```python
from build123d import *

# Parameters (mm, degrees)
BOSS_EXTRUDE1_DEPTH = 9.525
SKETCH2_R           = 10
BOSS_EXTRUDE2_DEPTH = 6.35
CUT_EXTRUDE1_REACH  = 36.757
SKETCH3_R           = 3.175
SKETCH4_R           = 3.175
CUT_EXTRUDE2_DEPTH  = 30.053883131


with BuildPart() as part:
    # Sketch1 → Boss-Extrude1 (new, symmetric)
    with BuildSketch(Plane.XY):
        Polygon((-9.525, 12.7), (-9.525, -12.7), (9.525, -12.7), (9.525, 12.7), (4.445, 12.7), (4.445, -7.62), (-4.445, -7.62), (-4.445, 12.7), align=None)
    extrude(amount=BOSS_EXTRUDE1_DEPTH, both=True)

    # Sketch2 → Boss-Extrude2 (add)
    with BuildSketch(Plane.XZ.offset(12.7)):
        with Locations(Location((0, 0, 0), (0, 0, 162.269593739))):
            Circle(SKETCH2_R)
    extrude(amount=BOSS_EXTRUDE2_DEPTH)

    # Sketch3 → Cut-Extrude1 (cut, up to next)
    with BuildSketch(Plane.XZ.offset(19.05), mode=Mode.PRIVATE) as cut_extrude1_sk1:
        Circle(SKETCH3_R)
    cut_extrude1_tool1 = extrude(cut_extrude1_sk1.sketch, amount=-CUT_EXTRUDE1_REACH, mode=Mode.PRIVATE) & part.part
    add(cut_extrude1_tool1.solids().sort_by_distance((0, -19.05, 0))[0], mode=Mode.SUBTRACT)

    # Sketch4 → Cut-Extrude2 (cut, through all)
    with BuildSketch(Plane(origin=(9.525, 0, 0), x_dir=(0, 0, -1), z_dir=(1, 0, 0))):
        with Locations((0, 3.175)):
            Circle(SKETCH4_R)
    extrude(amount=-CUT_EXTRUDE2_DEPTH, mode=Mode.SUBTRACT)


solid = part.part
```
The listing builds one solid part. Answer for the finished solid, in the listing's coordinates (mm). A direction names the side the tool comes from. Round coordinates to 2 decimals unless told otherwise and drop trailing zeros. Order: outer loops, then holes, each group sorted by start corner. A loop starts at its lowest first (then second) coordinate and runs counter-clockwise, first axis right, second up. Notation, with made-up numbers: (67, 76) - (86, 76) arc R33 ccw to (86, 110) - close; hole circle Ø2 at (5.5, 21). An arc over 180 degrees is marked (long way). Put each result on its own line as item: value. Start each with the question number.
(1) Given P1, Ø1.5, axis at y = -10, z = 1.5, coming from the -X side (3 decimals); P2, Ø4, axis at x = 1, z = 1, coming from the -Y side; P3, Ø12, axis at x = 0.5, y = -3, coming from the -Z side (3 decimals); P4, Ø10, axis at y = 5, z = 3.5, coming from the +X side (3 decimals), each flat-ended and moving along its own axis, determine where each tip first touches the part or whether it passes through.
(2) Find section C-C (y = -7). Give the vertices of the cut face in (x, z) (3 decimals), plus the area to 3 significant figures.
(3) Determine the mould class of faces 5 (the cylindrical face through (-0.69, -13.42, -3.1)), 6 (the flat face through (-4.445, 0, 2)), 7 (the flat face through (0, -8, -9.525)) for opening direction Z: released by +Z, released by -Z, zero draft, split by the parting line, or undercut.
(4) Find section A-A (x = 0). Give the vertices of the cut face in (y, z) (3 decimals), plus the area to 3 significant figures.
(5) For faces 1 (the flat face through (-3, -7.62, 2)), 2 (the flat face through (8, -12.7, -8)), 3 (the flat face through (8, -12.7, 8)), 4 (the flat face through (-8, -12.7, -8)), determine the directions among +Z, -Z, +X, -X, +Y, -Y from which every point of the face is accessible in a straight line to the end or side of a thin tool.
(6) Straight lines are drawn through the part: probe 1 along X at (y, z) = (-3, -3.5) (3 decimals); probe 2 along Y at (x, z) = (-7.85, 0); probe 3 along Y at (x, z) = (-0.5, -3.5). For each, find the intervals that lie inside material, in ascending order. Write a range as from..to.
(7) Find section B-B (z = 0). Give the vertices of the cut face in (x, y) (3 decimals), plus the area to 3 significant figures.
(8) Find section D-D (x = 5.5). Give the vertices of the cut face in (y, z) (3 decimals).
Reply:
1. P1: x = -9.525
1. P2: y = -19.05
1. P3: z = -9.525
1. P4: x = 9.525
2. outline: (-9.525, -9.525) - (-4.445, -9.525) - (-4.445, 9.525) - (-9.525, 9.525) - close; (4.445, -9.525) - (9.525, -9.525) - (9.525, 9.525) - (4.445, 9.525) - close
2. area: 194 mm^2
3. face 5: undercut
3. face 6: zero draft
3. face 7: released by -Z
4. outline: (-19.05, -10) - (-12.7, -10) - (-12.7, -9.525) - (-7.62, -9.525) - (-7.62, -3.175) - (-19.05, -3.175) - close; (-19.05, 3.175) - (-7.62, 3.175) - (-7.62, 9.525) - (-12.7, 9.525) - (-12.7, 10) - (-19.05, 10) - close
4. area: 151 mm^2
5. face 1: +Z, -Z, +Y
5. face 2: -Z, +X, -Y
5. face 3: +Z, +X, -Y
5. face 4: -Z, -X, -Y
6. probe 1: -9.525..-4.445, 4.445..9.525
6. probe 2: -19.05..0, 6.35..12.7
6. probe 3: -19.05..-7.62
7. outline: (-10, -19.05) - (-3.175, -19.05) - (-3.175, -7.62) - (-4.445, -7.62) - (-4.445, 0) - (-9.525, 0) - (-9.525, -12.7) - (-10, -12.7) - close; (-9.525, 6.35) - (-4.445, 6.35) - (-4.445, 12.7) - (-9.525, 12.7) - close; (3.175, -19.05) - (10, -19.05) - (10, -12.7) - (9.525, -12.7) - (9.525, 0) - (4.445, 0) - (4.445, -7.62) - (3.175, -7.62) - close; (4.445, 6.35) - (9.525, 6.35) - (9.525, 12.7) - (4.445, 12.7) - close
7. area: 293 mm^2
8. outline: (-19.05, -8.352) - (-12.7, -8.352) - (-12.7, -9.525) - (12.7, -9.525) - (12.7, 9.525) - (-12.7, 9.525) - (-12.7, 8.352) - (-19.05, 8.352) - close; hole circle Ø6.35 at (3.175, 0)
